```python
from build123d import *

# Parameters (mm, degrees)
F1_DEPTH = 3
F3_DEPTH = 3.001
F5_DEPTH = 3.001
F7_D     = 1


with BuildPart() as f1:
    # F0 (on Top) → F1 (new body)
    with BuildSketch(Plane.XY):
        with BuildLine():
            ThreePointArc((0, 3), (0.87868, 0.87868), (3, 0))
            Line((3, 0), (67, 0))
            ThreePointArc((67, 0), (69.12132, 0.87868), (70, 3))
            Line((70, 3), (70, 39))
            ThreePointArc((70, 39), (69.12132, 41.12132), (67, 42))
            Line((67, 42), (3, 42))
            ThreePointArc((3, 42), (0.87868, 41.12132), (0, 39))
            Line((0, 39), (0, 3))
        make_face()
    extrude(amount=F1_DEPTH)

    # F2 (on face) → F3 (cut, through all)
    with BuildSketch(Plane.XY.offset(3)):
        with BuildLine():
            Line((57.25, 10), (12.75, 10))
            ThreePointArc((12.75, 10), (11.335786, 9.414214), (10.75, 8))
            Line((10.75, 8), (10.75, 0))
            Line((10.75, 0), (59.25, 0))
            Line((59.25, 0), (59.25, 8))
            ThreePointArc((59.25, 8), (58.664214, 9.414214), (57.25, 10))
        make_face()
    extrude(amount=-F3_DEPTH, mode=Mode.SUBTRACT)

    # F4 (on face) → F5 (cut, through all)
    with BuildSketch(Plane.XY.offset(3)):
        Polygon((38.95, 37), (38.95, 42), (18.4, 42), (11.45, 42), (11.45, 34), (20.45, 34), (20.45, 35.4), (27.95, 35.4), (27.95, 37), align=None)
    extrude(amount=-F5_DEPTH, mode=Mode.SUBTRACT)

    # F7 (through all)
    with Locations(Plane.XY.offset(3)):
        with Locations((4, 38), (66, 38), (66, 4), (4, 4)):
            Hole(F7_D / 2)


solid = f1.part
```
The listing builds one solid part. Answer for the finished solid, in the listing's coordinates (mm). A direction names the side the tool comes from. Round coordinates to 2 decimals unless told otherwise and drop trailing zeros. Loops run counter-clockwise (first coordinate to the right, second up) from the corner with the lowest first, then second, coordinate; pieces in that order, holes last. Notation, with made-up numbers: (66.25, 76) - (116.25, 76) arc R22 cw to (116.25, 100) - close; hole circle Ø8 at (-6.75, 46.5). An arc over 180 degrees is marked (long way). Return JSON: item names as keys, results as strings. Group by question number.
1. Each of these flat-tipped pins is pushed along its axis until it touches: P1, Ø0.9, axis at x = 24.5, z = 1, coming from the +Y side; P2, Ø1.5, axis at x = 25, z = 2, coming from the -Y side; P3, Ø1.5, axis at x = 31, z = 1.5, coming from the +Y side. Where does it stop, or does it pass through?
2. Consider probe 1 along X at (y, z) = (38, 0.95); probe 2 along Y at (x, z) = (4, 1.85); probe 3 along X at (y, z) = (36, 2.45). Determine where each line is inside the solid, lowest interval first.
3. The part is cut by section B-B on x = 31. Determine the outline of the cut face in (y, z).
4. The part is cut by section C-C on x = 54.5. Determine the outline of the cut face in (y, z).
5. Which of the six approach directions +Z, -Z, +X, -X, +Y, -Y give full straight-line access (tool end or side, diameter ignored) to faces 1 (the flat face through (10.75, 4, 2)), 2 (the cylindrical face through (69.1, 0.86, 1.48)), 3 (the flat face through (16, 34, 2))?
6. The part is cut by section A-A on z = 1.5. Determine the outline of the cut face in (x, y), then the cut area to 3 significant figures.
7. The mould has two halves that part along X. Classify faces 4 (the flat face through (53, 42, 1)), 5 (the cylindrical face through (11.35, 9.43, 1.52)), 6 (the cylindrical face through (69.14, 41.1, 1.48)), 7 (the flat face through (0, 21, 1)): pulls with the +X half, pulls with the -X half, needs draft (parallel to the pull), parting line crosses it, or undercut.
Resolved:
{
 "1": {"P1": "stops at y = 35.4", "P2": "stops at y = 10", "P3": "stops at y = 37"},
 "2": {"probe 1": "x = 0 to 3.5, 4.5 to 11.45, 38.95 to 65.5, 66.5 to 70", "probe 2": "y = 0 to 3.5, 4.5 to 37.5, 38.5 to 42", "probe 3": "x = 0 to 11.45, 27.95 to 70"},
 "3": {"outline": "(10, 0) - (37, 0) - (37, 3) - (10, 3) - close"},
 "4": {"outline": "(10, 0) - (42, 0) - (42, 3) - (10, 3) - close"},
 "5": {"face 1": "+Z, -Z, -Y", "face 2": "+Z, -Z, +X, -Y", "face 3": "+Z, -Z, +Y"},
 "6": {"outline": "(0, 3) arc R3 ccw to (3, 0) - (10.75, 0) - (10.75, 8) arc R2 cw to (12.75, 10) - (57.25, 10) arc R2 cw to (59.25, 8) - (59.25, 0) - (67, 0) arc R3 ccw to (70, 3) - (70, 39) arc R3 ccw to (67, 42) - (38.95, 42) - (38.95, 37) - (27.95, 37) - (27.95, 35.4) - (20.45, 35.4) - (20.45, 34) - (11.45, 34) - (11.45, 42) - (3, 42) arc R3 ccw to (0, 39) - close; hole circle Ø1 at (4, 4); hole circle Ø1 at (4, 38); hole circle Ø1 at (66, 4); hole circle Ø1 at (66, 38)", "area": "2,270 mm²"},
 "7": {"face 4": "needs draft", "face 5": "undercut", "face 6": "pulls with the +X half", "face 7": "pulls with the -X half"}
}
